Autodesk Inventor part; units mm, degrees
ref_plane "YZ Plane" through (0, 0, 0) normal (1, 0, 0) x (0, 1, 0)
ref_plane "XZ Plane" through (0, 0, 0) normal (0, 1, 0) x (-1, 0, 0)
ref_plane "XY Plane" through (0, 0, 0) normal (0, 0, 1) x (1, 0, 0)
sketch "Sketch1" plane through (0, 0, 0) normal (0, 0, 1) x (1, 0, 0)
  line L0 (7.5, -1.5) -> (-7.5, -1.5)
  arc A0 (7.5, -1.5) -> (7.5, 1.5) centre (7.3777, 0) ccw
  line L1 (0, -2.1) -> (0, 2.1) construction
  arc A1 (-7.5, 1.5) -> (-7.5, -1.5) centre (-7.3777, 0) ccw
  line L2 (-12.4357, 0) -> (12.4357, 0) construction
  line L3 (7.5, 1.5) -> (-7.5, 1.5)
  point P0 (0, 0)
  point P1 (0, 1.5)
  dimension "d0" = 15
  dimension "d1" = 3
extrude "Extrusion1" add sketch "Sketch1" along normal blind 4.95
sketch "Sketch2" plane through (0, 0, 4.95) normal (0, 0, 1) x (1, 0, 0)
  line L0 (-12.5, 5) -> (12.5, 5)
  line L1 (12.5, 5) -> (12.5, -5)
  line L2 (12.5, -5) -> (-12.5, -5)
  line L3 (-12.5, -5) -> (-12.5, 5)
  point P0 (0, 0)
  point P1 (0, 5)
  point P2 (12.5, 0)
  dimension "d4" = 25
  dimension "d5" = 10
extrude "Extrusion2" add sketch "Sketch2" along normal blind 3
sketch "Sketch3" plane through (0, 0, 0) normal (0, 0, -1) x (-1, 0, 0)
  line L0 (-0.8, 1.5) -> (-0.8, -1.5)
  line L1 (-0.8, -1.5) -> (7.5, -1.5)
  arc A0 (7.5, -1.5) -> (7.5, 1.5) centre (7.3777, 0) ccw
  line L2 (7.5, 1.5) -> (-0.8, 1.5)
  line L3 (7.5, 1.5) -> (-7.5, 1.5)
  point P0 (0, 0)
extrude "Extrusion3" add sketch "Sketch3" along normal blind 14
sketch "Sketch5" plane through (-7.5, 1.5, 4.95) normal (0, 1, 0) x (1, 0, 0)
  circle A0 centre (3.35, 8.35) radius 1.25
  circle A1 centre (3.35, 15.374) radius 1.25
  line L0 (-5, 0) -> (-5, -3)
  line L1 (-5, 0) -> (20, 0)
  point P0 (7.5, 4.95)
  dimension "d18" = 2.5
  dimension "d19" = 8.35
  dimension "d20" = 8.35
  dimension "d21" = 7.024
extrude "Extrusion5" cut sketch "Sketch5" against normal through all
fillet "Fillet1" radius 2 6 edges at (0.8, 0, 0) (0.8, 0, -14) (-12.5, 5, 6.45) (-12.5, -5, 6.45) (12.5, -5, 6.45) (12.5, 5, 6.45)
properties part number "StartSupport"
Can you work these out from the model? Positions are in its coordinate system, mm. A direction names the side the tool comes from. Round coordinates to 2 decimals unless told otherwise and drop trailing zeros. Loops run counter-clockwise (first coordinate to the right, second up) from the corner with the lowest first, then second, coordinate; pieces in that order, holes last. Notation, with made-up numbers: (-5.75, 3) -> (-0.75, 3) arc R36 ccw to (-0.75, 39) -> close; hole circle Ø9 at (67.25, 51.5). An arc over 180 degrees is marked (long way). Answer in a Markdown table with one row per item.
Item 1: Will these pins go through, and if not, where does the flat tip stop? P1, Ø1.5, axis at x = 1, z = 4, coming from the +Y side; P2, Ø2, axis at y = 1.5, z = -11, coming from the +X side; P3, Ø12, axis at x = -3, z = -4, coming from the -Y side.
Answer block:
| item | result |
|---|---|
| P1 | y = 1.5 |
| P2 | x = 0.8 |
| P3 | y = -1.5 |
Item 2: On a 3-axis mill with a long thin cutter (end or side, diameter ignored), from which of +Z, -Z, +X, -X, +Y, -Y can I reach the whole of each face in a straight line? I mean faces 1 (the flat face through (12.5, 0, 6)), 2 (the cylindrical face through (-8.882, 0.031, -4.392)), 3 (the flat face through (-2, -1.5, -2)), 4 (the flat face through (-2, 1.5, -2)), 5 (the flat face through (6, 0, 0)). Say none if no direction works.
Answer block:
| item | result |
|---|---|
| face 1 | +Z, -Z, +X, +Y, -Y |
| face 2 | -Z, -X |
| face 3 | -Z, +X, -X, -Y |
| face 4 | -Z, +X, -X, +Y |
| face 5 | -Z, +X, +Y, -Y |
Item 3: We'd pull the mould along Z, two halves only. Please class faces 6 (the cylindrical face through (8.882, 0.031, 2.44)), 7 (the cylindrical face through (1.4, -0.02, -0.57)), 8 (the flat face through (0, 0, 7.95)), 9 (the cylindrical face through (-2.958, 0.021, -10.799)): released by +Z, released by -Z, zero draft, split by the parting line, or undercut.
Answer block:
| item | result |
|---|---|
| face 6 | zero draft |
| face 7 | released by -Z |
| face 8 | released by +Z |
| face 9 | undercut |
Item 4: If I drill on probe 1 along Z at (x, y) = (-4.15, -0.3); probe 2 along X at (y, z) = (0.15, -3.4); probe 3 along Y at (x, z) = (-2.5, -9.5), over which ranges is the centre line in solid material (lowest first)?
Answer block:
| item | result |
|---|---|
| probe 1 | -14 to -11.67, -9.17 to -4.65, -2.15 to 7.95 |
| probe 2 | -8.88 to -5.4, -2.9 to 0.8 |
| probe 3 | -1.5 to 1.5 |
Item 5: Suppose I cut it at D-D, the plane y = 0.75. List the corners of the cut face in (x, z) for me, plus the area to 3 significant figures.
Answer block:
| item | result |
|---|---|
| outline | (-12.5, 4.95) -> (-8.68, 4.95) -> (-8.68, -14) -> (-1.2, -14) arc R2 ccw to (0.8, -12) -> (0.8, -2) arc R2 cw to (2.8, 0) -> (8.68, 0) -> (8.68, 4.95) -> (12.5, 4.95) -> (12.5, 7.95) -> (-12.5, 7.95) -> close; hole circle Ø2.5 at (-4.15, -10.42); hole circle Ø2.5 at (-4.15, -3.4) |
| area | 284 mm² |
Item 6: Suppose I cut it at B-B, the plane x = -4.15. List the corners of the cut face in (y, z) for me.
Answer block:
| item | result |
|---|---|
| outline | (-5, 4.95) -> (-1.5, 4.95) -> (-1.5, -2.15) -> (1.5, -2.15) -> (1.5, 4.95) -> (5, 4.95) -> (5, 7.95) -> (-5, 7.95) -> close; (-1.5, -14) -> (1.5, -14) -> (1.5, -11.67) -> (-1.5, -11.67) -> close; (-1.5, -9.17) -> (1.5, -9.17) -> (1.5, -4.65) -> (-1.5, -4.65) -> close |
Item 7: Suppose I cut it at C-C, the plane x = 4.5. List the corners of the cut face in (y, z) for me, plus the area to 4 significant figures.
Answer block:
| item | result |
|---|---|
| outline | (-5, 4.95) -> (-1.5, 4.95) -> (-1.5, 0) -> (1.5, 0) -> (1.5, 4.95) -> (5, 4.95) -> (5, 7.95) -> (-5, 7.95) -> close |
| area | 44.85 mm² |
